For this review, take the finished solid that the model builds, in its own axes (mm). Face numbers are marked on the shaded views. Coordinates: 2 decimals unless noted, no trailing zeros. Loops run counter-clockwise (first coordinate to the right, second up) from the corner with the lowest first, then second, coordinate; pieces in that order, holes last. Notation, with made-up numbers: (80.5, -8.5) -> (98.5, -8.5) arc R10 cw to (98.5, 3.5) -> close; hole circle Ø2 at (70, 29). An arc over 180 degrees is marked (long way). Answer in a Markdown table with one row per item.
from build123d import *

# Parameters (mm, degrees)
CUT_EXTRUDE_1_DEPTH      = 64.231655884
CUT_EXTRUDE_1_DEPTH_BACK = 64.231655884
SKETCH_1_W               = 40
SKETCH_1_H               = 9


# Read off the part's stored shape, not the designer's step: Кнопка канцелярская
with BuildPart() as part:
    # Other 325 outline → Other 325 (revolve)
    with BuildSketch(Plane(origin=(0, 17.801844428, 11.6152978), x_dir=(0, 1, 0), z_dir=(0, 0, -1))):
        with BuildLine():
            Line((0, -32.931249855), (0, -44.931249855))
            Line((0, -44.931249855), (4.5, -44.931249855))
            ThreePointArc((4.5, -44.931249855), (3.767766953, -43.163482902), (2, -42.431249855))
            Line((2, -42.431249855), (1.5, -34.931249855))
            Line((1.5, -34.931249855), (3.500000006, -33.931249858))
            ThreePointArc((3.500000006, -33.931249858), (1.820027476, -33.186153702), (0, -32.931249855))
        make_face()
    revolve(axis=Axis((0, 17.801844428, 11.6152978), (1, 0, 0)))


with BuildPart() as body_2:
    # Other 325 2 outline → Other 325 2 (revolve)
    with BuildSketch(Plane(origin=(0, 17.801844428, 11.6152978), x_dir=(0, 1, 0), z_dir=(0, 0, -1))):
        with BuildLine():
            Line((0.6, -44.931249855), (0, -44.931249855))
            Line((0, -44.931249855), (0, -56.931249855))
            Line((0, -56.931249855), (0.489363529, -53.66882633))
            ThreePointArc((0.489363529, -53.66882633), (0.572302525, -52.929184099), (0.6, -52.185421801))
            Line((0.6, -52.185421801), (0.6, -44.931249855))
        make_face()
    revolve(axis=Axis((0, 17.801844428, 11.6152978), (1, 0, 0)))


with BuildPart() as cut_extrude_1_tool:
    # Эскиз1 → Вырез-Вытянуть1 (new, two sides: drawn at the far end of the back side and taken through both)
    with BuildSketch(Plane.XY.offset(-CUT_EXTRUDE_1_DEPTH_BACK)):
        with Locations((-56.931249855, 17.801844428)):
            Rectangle(SKETCH_1_W, SKETCH_1_H)
    extrude(amount=CUT_EXTRUDE_1_DEPTH + CUT_EXTRUDE_1_DEPTH_BACK)


with BuildPart() as part_1:
    add(part.part)

    # Вырез-Вытянуть1: cut by cut_extrude_1_tool
    add(cut_extrude_1_tool.part, mode=Mode.SUBTRACT)

    # Эскиз2 → Повернуть1 (revolve)
    with BuildSketch(Plane(origin=(-44.931249855, 17.801844428, 11.6152978), x_dir=(1, 0, 0), z_dir=(0, 0, 1)), mode=Mode.PRIVATE) as revolve_1_sk:
        with BuildLine():
            Line((8, 0), (8, 2))
            ThreePointArc((8, 2), (7.5, 2.5), (7, 2))
            Line((7, 2), (7, 0))
            Line((7, 0), (8, 0))
        make_face()
    revolve(revolve_1_sk.sketch.rotate(Axis((-36.931249855, 17.801844428, 11.6152978), (-1, 0, 0)), 90), axis=Axis((-36.931249855, 17.801844428, 11.6152978), (-1, 0, 0)))


with BuildPart() as body_2_1:
    add(body_2.part)

    # Вырез-Вытянуть1: cut by cut_extrude_1_tool
    add(cut_extrude_1_tool.part, mode=Mode.SUBTRACT)


solid = part_1.part
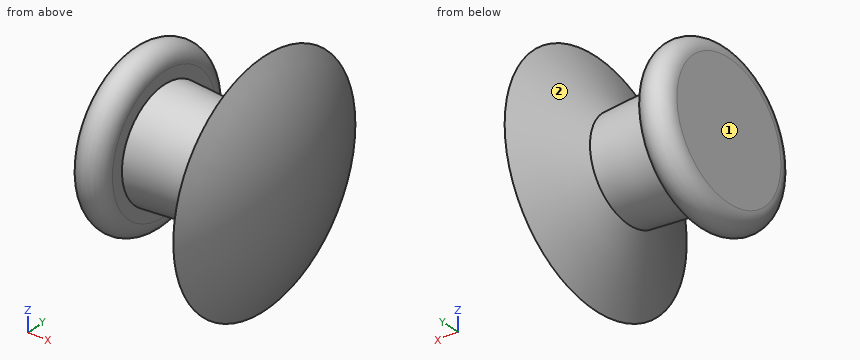
Item 1: For L1, parallel to X at y = 18.75, z = 9.5; L2, parallel to X at y = 18, z = 13.5; L3, parallel to Z at x = -37.4, y = 18.5, list the stretches that pass through material, from the lowest coordinate up.
Worked answers:
| item | result |
|---|---|
| L1 | -37.82 to -37.05, -34.52 to -33.35 |
| L2 | -37.93 to -36.93, -34.73 to -33.21 |
| L3 | 9.22 to 14.01 |
Item 2: Take a section at B-B, the plane x = -36.75. State the section outline as (y, z) points, and give its area (3 significant figures).
Worked answers:
| item | result |
|---|---|
| outline | circle Ø3.24 at (17.8, 11.62) |
| area | 8.26 mm² |
Item 3: Take a section at A-A, the plane x = -35.3. State the section outline as (y, z) points, and give its area (3 significant figures).
Worked answers:
| item | result |
|---|---|
| outline | circle Ø3.05 at (17.8, 11.62) |
| area | 7.30 mm² |
Item 4: Insertion check: pin 1 (1.5 mm diameter, centred on x = -37, y = 19.5, fed in from +Z); pin 2 (2 mm diameter, centred on x = -35, y = 17.5, fed in from +Z); pin 3 (3 mm diameter, centred on x = -35.5, y = 16, fed in from -Z). Each pin has a flat end and moves straight along its axis. Give the tip position at first contact, or say it passes through.
Worked answers:
| item | result |
|---|---|
| pin 1 | z = 13.88 |
| pin 2 | z = 14.97 |
| pin 3 | z = 8.67 |
Item 5: The part is to be moulded in two halves that separate along X. For the marked faces 1 and 2, say which applies: +X half, -X half, draft (parallel to the pull), parting line (faces both ways), or undercut.
Worked answers:
| item | result |
|---|---|
| face 1 | -X half |
| face 2 | undercut |
